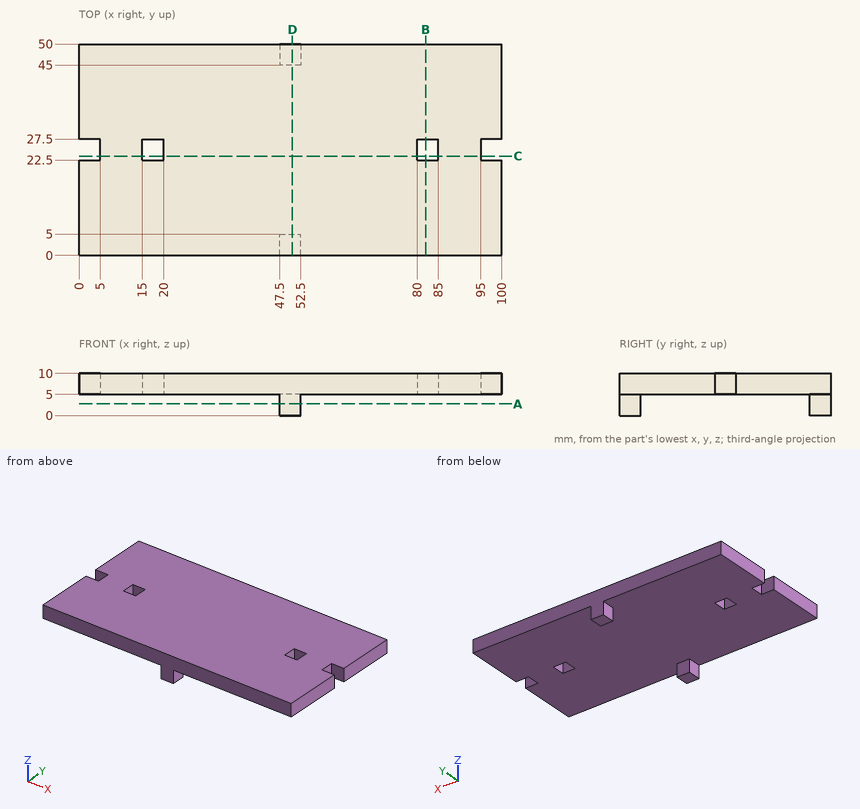
Source: three-view drawing plus pictorial views. Frame: mm from the lowest corner of the part. Round coordinates to 2 decimals unless told otherwise and drop trailing zeros. Loops run counter-clockwise (first coordinate to the right, second up) from the corner with the lowest first, then second, coordinate; pieces in that order, holes last. Notation, with made-up numbers: M -33.5,-25.75 L 6.5,-25.75 A21 cw 6.5,3.25 Z; hole C -33.5,-2 d2. An arc over 180 degrees is marked long. Put each result on its own line as item: value.
(1) Section A-A, the plane z = 2.75. Return loops of the section in (x, y), and give its area (3 significant figures).
Solutions:
outline: M 47.5,0 L 52.5,0 L 52.5,5 L 47.5,5 Z; M 47.5,45 L 52.5,45 L 52.5,50 L 47.5,50 Z
area: 50.0 mm²
(2) Section B-B, the plane x = 82. Return loops of the section in (y, z), and give its area (3 significant figures).
Solutions:
outline: M 0,5 L 22.5,5 L 22.5,10 L 0,10 Z; M 27.5,5 L 50,5 L 50,10 L 27.5,10 Z
area: 225 mm²
(3) Section D-D, the plane x = 50.5. Return loops of the section in (y, z), and give its area (3 significant figures).
Solutions:
outline: M 0,0 L 5,0 L 5,5 L 45,5 L 45,0 L 50,0 L 50,10 L 0,10 Z
area: 300 mm²
(4) Section C-C, the plane y = 23.5. Return loops of the section in (x, z), and give its area (3 significant figures).
Solutions:
outline: M 5,5 L 15,5 L 15,10 L 5,10 Z; M 20,5 L 80,5 L 80,10 L 20,10 Z; M 85,5 L 95,5 L 95,10 L 85,10 Z
area: 400 mm²
(5) First-contact query: pin 1 (1.5 mm diameter, centred on y = 25, z = 6.5, fed in from -X); pin 2 (2.5 mm diameter, centred on y = 48.5, z = 1.5, fed in from -X); pin 3 (4 mm diameter, centred on x = 74.5, y = 30.5, fed in from -Z). Flat tips, straight axial feed; report the tip coordinate or a pass-through.
Solutions:
pin 1: x = 5
pin 2: x = 47.5
pin 3: z = 5
(6) Ray query, line 1 (Y direction, x = 82, z = 9); line 2 (Y direction, x = 49, z = 0.5); line 3 (Z direction, x = 56.5, y = 26). Return the intervals inside material, ascending. Write a range as [from, to].
Solutions:
line 1: [0, 22.5], [27.5, 50]
line 2: [0, 5], [45, 50]
line 3: [5, 10]
